```python
from build123d import *

# Parameters (mm, degrees)
F1_DEPTH = 25
F3_R     = 5


# Not quite as in the source:
# - a feature names something its author has since deleted; it is built from what else it names


with BuildPart() as f1:
    # F0 (on Front) → F1 (new body)
    with BuildSketch(Plane.XZ):
        with BuildLine():
            ThreePointArc((11.8972236274, -13.5987717306), (19.6369586065, -18.770230883), (17.4821764595, -9.7146027319))
            ThreePointArc((17.4821764595, -9.7146027319), (18.3784296837, 7.8888099459), (5, 19.364916731))
            Line((5, 19.364916731), (5, 20.2805753797))
            Line((5, 20.2805753797), (0, 20.2805753797))
            Line((0, 20.2805753797), (0, 20))
            Line((0, 20), (0, 15))
            ThreePointArc((0, 15), (12.7749432268, 7.86135011), (13.3904401788, -6.7598899265))
            Line((13.3904401788, -6.7598899265), (11.8972236274, -13.5987717306))
        make_face()
    extrude(amount=F1_DEPTH)

    # F2: F1 across plane


with BuildPart() as f1_1:
    add(f1.part)
    add(f1.part.mirror(Plane.YZ))

    # F3
    f3_edges = [f1_1.edges().sort_by_distance(p)[0] for p in [
        (-17.482176, -12.5, -9.714603),
        (17.482176, -12.5, -9.714603),
        (0, -25, 20.280575),
        (0, 0, 20.280575),
    ]]
    fillet(f3_edges, radius=F3_R)


solid = f1_1.part
```
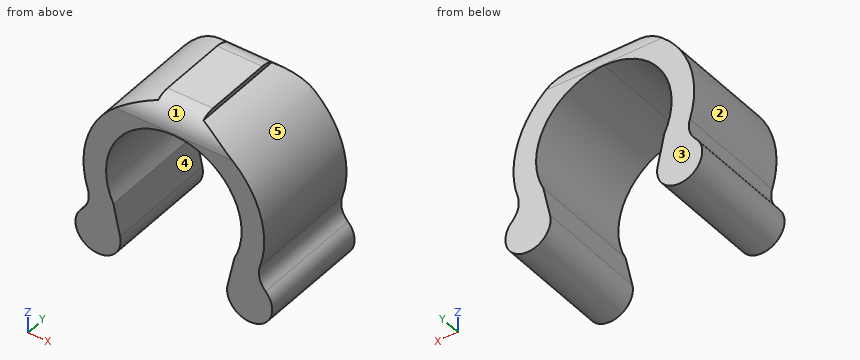
Model file for the job. Use its own axes, mm. Face numbers are marked on the shaded views. A direction names the side the tool comes from. Round coordinates to 2 decimals unless told otherwise and drop trailing zeros. Write each loop counter-clockwise with the first axis right and the second up, starting at its lowest first coordinate (ties: lowest second). Pieces come first, ordered by that corner, then holes. Notation, with made-up numbers: (-22.5, -35) - (6.5, -35) arc R17 cw to (6.5, -26) - close; hole circle Ø11 at (0.25, 63.25). An arc over 180 degrees is marked (long way). Use CSV: the item, a comma, the result in double quotes. Start each with the question number.
Item 1: Drill centre lines: L1, parallel to X at y = -7.5, z = -15; L2, parallel to X at y = -20.75, z = -12.5; L3, parallel to Z at x = 0, y = -17.5. Where is each one in solid material? Low to high. Write a range as [from, to].
Item 2: Tool access for the marked faces 4 and 5: list every direction of +Z, -Z, +X, -X, +Y, -Y with a clear straight run to the whole face (end or side of a thin tool).
Item 3: Pin check, flat tips, straight feed: P1, Ø2, axis at y = -10, z = 15.5, coming from the +X side (3 decimals); P2, Ø4, axis at y = -18.5, z = 4, coming from the -X side; P3, Ø4, axis at y = -21.5, z = 9, coming from the -X side (3 decimals); P4, Ø8, axis at x = -16, z = 13, coming from the +Y side. Stop position of each tip, or through.
Item 4: Band-saw the part on C-C (z = 13). Write the cut outline in (x, y).
Item 5: Band-saw the part on D-D (x = 3). Write the cut outline in (y, z), and give its area (3 significant figures).
Item 6: Band-saw the part on A-A (z = 1). Write the cut outline in (x, y).
Item 7: Two-plate mould, pull along Z, no slides. Class the marked faces 1, 2 and 3: released by +Z, released by -Z, zero draft, split by the parting line, or undercut.
Item 8: Band-saw the part on B-B (x = -3.5). Write the cut outline in (y, z).
Checked values:
1,L1,"x = [-21.77, -11.79], [11.79, 21.77]"
1,L2,"x = [-21.29, -12.14], [12.14, 21.29]"
1,L3,"z = [15, 20.28]"
2,face 4,"+Y, -Y"
2,face 5,"+X, +Y, -Y"
3,P1,"stops at x = 13.775"
3,P2,"stops at x = -19.9"
3,P3,"stops at x = -18.735"
3,P4,"stops at y = 0"
4,outline,"(-15.2, -25) - (-7.48, -25) - (-7.48, 0) - (-15.2, 0) - close; (7.48, -25) - (15.2, -25) - (15.2, 0) - (7.48, 0) - close"
5,outline,"(-25, 14.7) - (0, 14.7) - (0, 15.28) arc R5 ccw to (-5, 20.28) - (-20, 20.28) arc R5 ccw to (-25, 15.28) - close"
5,area,"129 mm²"
6,outline,"(-19.97, -25) - (-14.97, -25) - (-14.97, 0) - (-19.97, 0) - close; (14.97, -25) - (19.97, -25) - (19.97, 0) - (14.97, 0) - close"
7,face 1,"released by +Z"
7,face 2,"undercut"
7,face 3,"zero draft"
8,outline,"(-25, 14.59) - (0, 14.59) - (0, 15.28) arc R5 ccw to (-5, 20.28) - (-20, 20.28) arc R5 ccw to (-25, 15.28) - close"
